Autodesk Inventor part; units mm, degrees
ref_plane "YZ Plane" through (0, 0, 0) normal (1, 0, 0) x (0, 1, 0)
ref_plane "XZ Plane" through (0, 0, 0) normal (0, 1, 0) x (-1, 0, 0)
ref_plane "XY Plane" through (0, 0, 0) normal (0, 0, 1) x (1, 0, 0)
sketch "Esboço1" plane through (0, 0, 0) normal (0, 0, 1) x (1, 0, 0)
  arc A0 (4, 2.4377) -> (-4, 2.4377) centre (0, 9.3659) ccw
  line L0 (9.25, -3.9341) -> (9.25, -10.6341)
  line L1 (-9.25, -10.6341) -> (-9.25, -3.9341)
  line L2 (4, -15.6341) -> (-4, -15.6341)
  line L3 (20, -15.6341) -> (-20, -15.6341)
  line L4 (-20, -15.6341) -> (-20, -10.6341)
  line L5 (20, -10.6341) -> (20, -15.6341)
  line L6 (7.6788, -3.9341) -> (9.25, -3.9341)
  line L7 (-9.25, -3.9341) -> (-7.6788, -3.9341)
  line L8 (9.25, -10.6341) -> (20, -10.6341)
  line L9 (-20, -10.6341) -> (-9.25, -10.6341)
  line L10 (-4, 2.4377) -> (-7.6788, -3.9341)
  line L11 (-17.4151, -20.798) -> (-22.4188, -29.4646)
  line L12 (17.4151, -20.798) -> (23.6527, -31.6017)
  line L13 (9.25, -15.6341) -> (4, -15.6341)
  line L14 (0, -15.6341) -> (-9.25, -15.6341)
  line L15 (4, 2.4377) -> (7.6788, -3.9341)
  dimension "d6" = 16
  dimension "d7" = 25
  dimension "d8" = 18.5
  dimension "d9" = 11.7
  dimension "d10" = 8
  dimension "d13" = 5
  dimension "d14" = 40
extrude "Extrusão1" add sketch "Esboço1" along normal blind 725
sketch "Esboço3" plane through (-20, -15.6341, 0) normal (0, -1, 0) x (1, 0, 0)
  line L0 (0, 725) -> (40, 725) construction
  line L1 (20, 725) -> (20, 0) construction
  line L2 (20, 705) -> (5, 705) construction
  line L3 (5, 705) -> (20, 705) construction
  line L4 (20, 705) -> (35, 705) construction
  circle A0 centre (5, 705) radius 2.75
  circle A1 centre (35, 705) radius 2.75
  line L5 (40, 0) -> (0, 0) construction
  dimension "d18" = 15
  dimension "d19" = 15
  dimension "d20" = 5.5
  dimension "d21" = 5.5
  dimension "d22" = 20
hole "Furo1" at (-15, -15.6341, 705) at (15, -15.6341, 705) direction (0, 1, 0) diameter 5.5 depth 8 tip angle 118
properties part number "SBR16_EIXO_X_2"
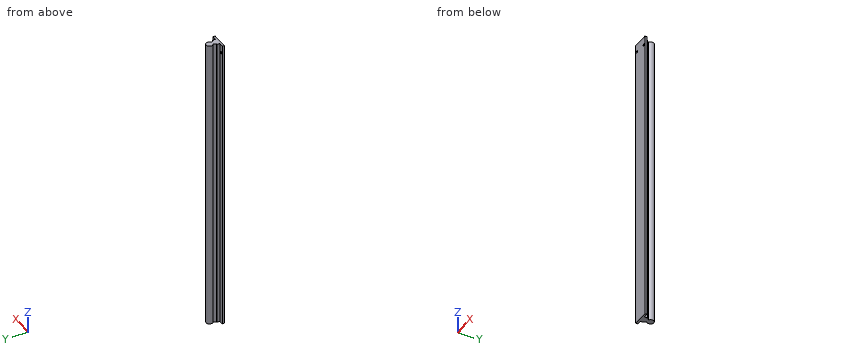
Work out the finished part from the listing and answer in its coordinate system (mm). Round coordinates to 2 decimals unless told otherwise and drop trailing zeros. Loops run counter-clockwise (first coordinate to the right, second up) from the corner with the lowest first, then second, coordinate; pieces in that order, holes last. Notation, with made-up numbers: (82, 3) -> (96, 3) arc R26 cw to (96, 28) -> close; hole circle Ø8 at (-31, 83). An arc over 180 degrees is marked (long way). Use one line per item in the form item = value.
(1) Straight lines are drawn through the part: line 1 (X direction, y = -14.5, z = 705); line 2 (Z direction, x = -15, y = -12.4); line 3 (Y direction, x = -1, z = 401). For each, find the intervals that lie inside material, in ascending order.
Answer list:
line_1 = -20 to -17.75, -12.25 to 12.25, 17.75 to 20
line_2 = 0 to 702.25, 707.75 to 725
line_3 = -15.63 to 17.3
(2) Flat-ended cylindrical pins translate along their axes: P1, Ø8.5, axis at x = 13, z = 362, coming from the +Y side; P2, Ø5, axis at y = 14, z = 638.5, coming from the +X side; P3, Ø5.5, axis at y = -6, z = 402, coming from the -X side. Find the tip coordinate at first contact, or state that the pin passes through.
Answer list:
P1 = -3.93
P2 = 7.71
P3 = -9.25
(3) Find section A-A on y = 10.5. Give the vertices of the cut face in (x, z), then the cut area to 3 significant figures.
Answer list:
outline = (-7.92, 0) -> (7.92, 0) -> (7.92, 725) -> (-7.92, 725) -> close
area = 11,500 mm2
